The listing builds one solid part. Answer for the finished solid, in the listing's coordinates (mm). A direction names the side the tool comes from. Round coordinates to 2 decimals unless told otherwise and drop trailing zeros. Loops run counter-clockwise (first coordinate to the right, second up) from the corner with the lowest first, then second, coordinate; pieces in that order, holes last. Notation, with made-up numbers: (63, 79.25) - (67, 79.25) arc R27 cw to (67, 97.25) - close; hole circle Ø10 at (49.25, 46.25). An arc over 180 degrees is marked (long way). One line per question, with ' | ' between items. Start each with the question number.
from build123d import *

# Parameters (mm, degrees)
F0_W     = 76.2
F0_H     = 50.8
F0_W_2   = 69.85
F0_H_2   = 44.45
F2_DEPTH = 345.44
F4_DEPTH = 50.801
F6_DEPTH = 50.801
F7_R     = 3.175


# Not quite as in the source:
# - a variable given as a bare number and used for a length is read in inches; the dataset says mm whatever the document's units were


with BuildPart() as f2:
    # F0 (on Front) → F2 (new body)
    with BuildSketch(Plane.XZ):
        Rectangle(F0_W, F0_H)
        Rectangle(F0_W_2, F0_H_2, mode=Mode.SUBTRACT)
    extrude(amount=F2_DEPTH)

    # F3 (on face) → F4 (cut, through all)
    with BuildSketch(Plane(origin=(0, 0, -25.4), x_dir=(1, 0, 0), z_dir=(0, 0, -1))):
        Polygon((38.1, 345.44), (-38.1, 345.44), (38.1, 269.24), align=None)
    extrude(amount=-F4_DEPTH, mode=Mode.SUBTRACT)

    # F5 (on face) → F6 (cut, through all)
    with BuildSketch(Plane(origin=(0, 0, -25.4), x_dir=(1, 0, 0), z_dir=(0, 0, -1))):
        Polygon((38.1, 76.2), (-38.1, 0), (38.1, 0), align=None)
    extrude(amount=-F6_DEPTH, mode=Mode.SUBTRACT)

    # F7
    f7_edges = [f2.edges().sort_by_distance(p)[0] for p in [
        (38.1, -172.72, -25.4),
        (-38.1, -172.72, -25.4),
        (-38.1, -172.72, 25.4),
        (38.1, -172.72, 25.4),
        (-34.925, -172.72, 22.225),
        (34.925, -172.72, 22.225),
        (-34.925, -172.72, -22.225),
        (34.925, -172.72, -22.225),
    ]]
    fillet(f7_edges, radius=F7_R)


solid = f2.part
(1) A tool of negligible diameter and unlimited length cuts with its end or side. For faces 5 (the flat face through (-34.925, -170, 0)), 6 (the flat face through (0, -170, -25.4)), from which of +Z, -Z, +X, -X, +Y, -Y can it reach the whole face along a straight path? Write none if from no direction.
(2) Find section C-C on y = -318.5. Write down the section's boundary in (x, z) (3 decimals), plus the area to 3 significant figures.
(3) Determine the mould class of faces 1 (the flat face through (0, -170, 25.4)), 2 (the flat face through (-38.1, -170, 0)), 3 (the flat face through (34.925, -171, 0)), 4 (the flat face through (38.1, -171, 0)) for opening direction X: pulls with the +X half, pulls with the -X half, needs draft (parallel to the pull), parting line crosses it, or undercut.
(4) Find section A-A on x = -23. Write down the section's boundary in (y, z) (3 decimals).
(5) Consider L1, parallel to X at y = -117.5, z = -5.5 (3 decimals); L2, parallel to Z at x = 5.5, y = -83 (3 decimals); L3, parallel to X at y = -331, z = -15.5 (3 decimals). Determine where each line is inside the solid, lowest interval first.
(6) Find section D-D on y = -108. Write down the section's boundary in (x, z) (3 decimals), plus the area to 3 significant figures.
(7) Find section B-B on z = 14.5. Write down the section's boundary in (x, y) (3 decimals).
Answer below:
1) face 5: +Y, -Y | face 6: -Z, +X, -X, +Y, -Y
2) outline: (-38.1, -22.225) arc R3.175 ccw to (-34.925, -25.4) - (-11.16, -25.4) - (-11.16, -22.225) - (-31.75, -22.225) arc R3.175 cw to (-34.925, -19.05) - (-34.925, 19.05) arc R3.175 cw to (-31.75, 22.225) - (-11.16, 22.225) - (-11.16, 25.4) - (-34.925, 25.4) arc R3.175 ccw to (-38.1, 22.225) - close | area: 312 mm2
3) face 1: needs draft | face 2: pulls with the -X half | face 3: undercut | face 4: pulls with the +X half
4) outline: (-330.34, -25.4) - (-15.1, -25.4) - (-15.1, -22.225) - (-330.34, -22.225) - close; (-330.34, 22.225) - (-15.1, 22.225) - (-15.1, 25.4) - (-330.34, 25.4) - close
5) L1: -38.1 to -34.925, 34.925 to 38.1 | L2: -25.4 to -22.225, 22.225 to 25.4 | L3: -38.1 to -34.925
6) outline: (-38.1, -22.225) arc R3.175 ccw to (-34.925, -25.4) - (34.925, -25.4) arc R3.175 ccw to (38.1, -22.225) - (38.1, 22.225) arc R3.175 ccw to (34.925, 25.4) - (-34.925, 25.4) arc R3.175 ccw to (-38.1, 22.225) - close; hole (-34.925, -19.05) arc R3.175 ccw to (-31.75, -22.225) - (31.75, -22.225) arc R3.175 ccw to (34.925, -19.05) - (34.925, 19.05) arc R3.175 ccw to (31.75, 22.225) - (-31.75, 22.225) arc R3.175 ccw to (-34.925, 19.05) - close | area: 766 mm2
7) outline: (-38.1, -345.44) - (-34.925, -342.265) - (-34.925, -3.175) - (-38.1, 0) - close; (34.925, -272.415) - (38.1, -269.24) - (38.1, -76.2) - (34.925, -73.025) - close
